Can you work these out from the model? Positions are in its coordinate system, mm. Face numbers are marked on the shaded views. A direction names the side the tool comes from. Give positions to 0.01 mm unless a question says otherwise; leave off trailing zeros. Write each loop counter-clockwise with the first axis right and the second up, starting at its lowest first coordinate (ties: lowest second). Pieces come first, ordered by that corner, then holes.
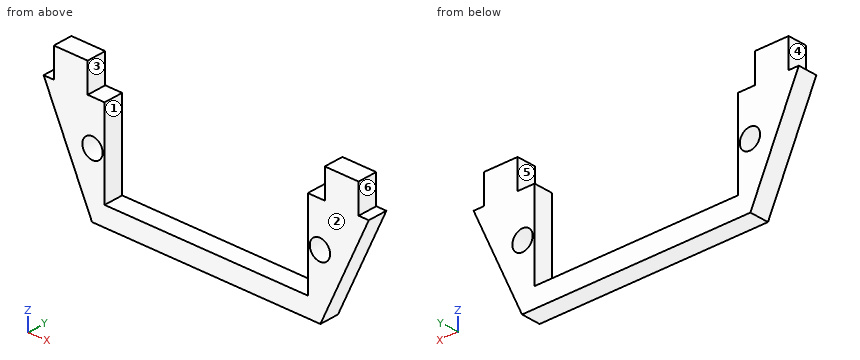
from build123d import *

# Parameters (mm, degrees)
CROQUIS1_R              = 1.05
SALIENTE_EXTRUIR1_DEPTH = 2


with BuildPart() as part:
    # Croquis1 → Saliente-Extruir1 (new body)
    with BuildSketch(Plane(origin=(0, 0, 0), x_dir=(1, 0, 0), z_dir=(0, 1, 0))):
        Polygon((-10.5, 0), (-10.5, 9), (10.5, 9), (10.5, 0), (12.25, 0), (12.25, -3), (15.75, -3), (15.75, 0), (16.8, 0), (11.8, 11), (-11.8, 11), (-16.8, 0), (-15.75, 0), (-15.75, -3), (-12.25, -3), (-12.25, 0), align=None)
        with Locations(Location((-11.75, 4.5, 0), (0, 0, 270))):
            Circle(CROQUIS1_R, mode=Mode.SUBTRACT)
        with Locations(Location((11.75, 4.5, 0), (0, 0, 270))):
            Circle(CROQUIS1_R, mode=Mode.SUBTRACT)
    extrude(amount=SALIENTE_EXTRUIR1_DEPTH)


solid = part.part
(1) If I drill on L1, parallel to X at y = 0.85, z = -4.5; L2, parallel to X at y = 1.35, z = -4.75; L3, parallel to Z at x = -4, y = 1.6, over which ranges is the centre line in solid material (lowest first)?
Returned:
L1: x = -14.75 to -12.8, -10.7 to -10.5, 10.5 to 10.7, 12.8 to 14.75
L2: x = -14.64 to -12.77, -10.73 to -10.5, 10.5 to 10.73, 12.77 to 14.64
L3: z = -11 to -9
(2) Imagine slicing it at B-B, the plane y = 1.7. Write out the boundary of the cut face in (x, z), plus the area to 3 significant figures.
Returned:
outline: (-16.8, 0) - (-11.8, -11) - (11.8, -11) - (16.8, 0) - (15.75, 0) - (15.75, 3) - (12.25, 3) - (12.25, 0) - (10.5, 0) - (10.5, -9) - (-10.5, -9) - (-10.5, 0) - (-12.25, 0) - (-12.25, 3) - (-15.75, 3) - (-15.75, 0) - close; hole circle Ø2.1 at (-11.75, -4.5); hole circle Ø2.1 at (11.75, -4.5)
area: 140 mm2
(3) Imagine slicing it at A-A, the plane z = 1.5. Write out the boundary of the cut face in (x, y).
Returned:
outline: (-15.75, 0) - (-12.25, 0) - (-12.25, 2) - (-15.75, 2) - close; (12.25, 0) - (15.75, 0) - (15.75, 2) - (12.25, 2) - close
(4) Will these pins go through, and if not, where does the flat tip stop? P1, Ø0.6, axis at y = 1, z = 2, coming from the +X side; P2, Ø1.3, axis at x = -11.75, z = -4.5, coming from the -Y side; P3, Ø0.6, axis at y = 0.5, z = -6.5, coming from the -X side; P4, Ø1, axis at y = 1, z = -2.5, coming from the +X side.
Returned:
P1: stops at x = 15.75
P2: passes through
P3: stops at x = -13.98
P4: stops at x = 15.89
(5) Imagine slicing it at D-D, the plane x = -3. Write out the boundary of the cut face in (y, z).
Returned:
outline: (0, -11) - (2, -11) - (2, -9) - (0, -9) - close
(6) If we mould it in two halves opening along X, with no side actions, what happens to the marked faces 3, 4, 5 and 6? For each: +X half, -X half, draft (parallel to the pull), parting line (faces both ways), or undercut.
Returned:
face 3: undercut
face 4: -X half
face 5: undercut
face 6: +X half
(7) For the marked faces 1 and 2, which set-ups out of +Z, -Z, +X, -X, +Y, -Y let a thin tool reach every point of the face, with its end or its side?
Returned:
face 1: +Z, +Y, -Y
face 2: +Z, -Z, +X, -X, -Y
(8) Imagine slicing it at C-C, the plane z = -4.5. Write out the boundary of the cut face in (x, y).
Returned:
outline: (-14.75, 0) - (-12.8, 0) - (-12.8, 2) - (-14.75, 2) - close; (-10.7, 0) - (-10.5, 0) - (-10.5, 2) - (-10.7, 2) - close; (10.5, 0) - (10.7, 0) - (10.7, 2) - (10.5, 2) - close; (12.8, 0) - (14.75, 0) - (14.75, 2) - (12.8, 2) - close
